Here's how the part is built. I have some questions about the finished solid (model axes, mm). A direction names the side the tool comes from. Round coordinates to 2 decimals unless told otherwise and drop trailing zeros. Write each loop counter-clockwise with the first axis right and the second up, starting at its lowest first coordinate (ties: lowest second). Pieces come first, ordered by that corner, then holes. Notation, with made-up numbers: (-30, 20.5) - (8, 20.5) arc R24 cw to (8, 57.5) - close; hole circle Ø4 at (-20.75, -32.75). An arc over 180 degrees is marked (long way). One line per question, with ' | ' between items. Start each with the question number.
(1) Will these pins go through, and if not, where does the flat tip stop? pin 1 (12 mm diameter, centred on y = -175, z = -100, fed in from +X); pin 2 (5 mm diameter, centred on x = 525, z = 23.5, fed in from +Y); pin 3 (6 mm diameter, centred on y = 211.5, z = -110.5, fed in from -X).
(2) For faces 4 (the cylindrical face through (910.575, -7.509, -23.846)), 5 (the cylindrical face through (572.9, -7.509, -23.846)), which set-ups out of +Z, -Z, +X, -X, +Y, -Y let a thin tool reach every point of the face, with its end or its side?
(3) If I drill on L1, parallel to X at y = 14.5, z = -144; L2, parallel to X at y = 77, z = -270.5; L3, parallel to Y at x = 754, z = 4.5, over which ranges is the centre line in solid material (lowest first)?
(4) Imagine slicing it at A-A (z = 84). Write out the boundary of the cut face in (x, y), plus the area to 3 significant figures.
(5) Thinking about a two-plate mould opening in X: for faces 1 (the cylindrical face through (184.875, -7.509, -23.846)), 2 (the flat face through (375, -62, 4)), 3 (the flat face through (725, -31, 2)), which applies, pulls with the +X half, pulls with the -X half, needs draft (parallel to the pull), parting line crosses it, or undercut?
(6) Imagine slicing it at D-D (z = -73.5). Write out the boundary of the cut face in (x, y).
(7) Imagine slicing it at B-B (x = 950.5). Write out the boundary of the cut face in (y, z), plus the area to 3 significant figures.
(8) Imagine slicing it at C-C (y = 240). Write out the boundary of the cut face in (x, z), plus the area to 3 significant figures.
Autodesk Inventor part; units mm, degrees
ref_plane "YZ Plane" through (0, 0, 0) normal (1, 0, 0) x (0, 1, 0)
ref_plane "XZ Plane" through (0, 0, 0) normal (0, 1, 0) x (-1, 0, 0)
ref_plane "XY Plane" through (0, 0, 0) normal (0, 0, 1) x (1, 0, 0)
sketch "Sketch1" plane through (0, 0, 0) normal (0, 1, 0) x (-1, 0, 0)
  line L0 (0, 0) -> (-400, 0) construction
  line L1 (-400, 0) -> (-750, 0)
  line L2 (-750, 0) -> (-1050, 0)
  line L3 (-400, 0) -> (-400, -300) construction
  line L4 (-400, -300) -> (-375, -300) construction
  line L5 (-375, -300) -> (-425, -300)
  line L6 (-425, -300) -> (-425, 0)
  line L7 (-425, 0) -> (-375, 0)
  line L8 (-375, 0) -> (-375, -300)
  line L9 (0, 0) -> (-1050, 0)
  line L10 (-1050, 0) -> (-1050, -25)
  line L11 (-1050, -25) -> (0, -25)
  line L12 (0, -25) -> (0, 0)
  arc A0 (0, -25) -> (25, 0) centre (0, 0) ccw
  line L13 (0, 0) -> (25, 0) construction
  line L14 (-750, 0) -> (-750, -150) construction
  line L15 (-750, -150) -> (-725, -150) construction
  line L16 (-725, -150) -> (-775, -150)
  line L17 (-775, -150) -> (-775, 0)
  line L18 (-775, 0) -> (-725, 0)
  line L19 (-725, 0) -> (-725, -150)
  arc A1 (-1075, 0) -> (-1050, -25) centre (-1050, 0) ccw
  line L20 (-1050, 0) -> (-1075, 0)
  line L21 (25, 0) -> (0, 0)
  point P0 (-775, -25)
  point P1 (-725, -25)
  point P2 (-425, -25)
  point P3 (-375, -25)
  dimension "d0" = 400
  dimension "d1" = 350
  dimension "d2" = 300
  dimension "d3" = 300
  dimension "d4" = 25
  dimension "d5" = 50
  dimension "d6" = 1050
  dimension "d7" = 25
  dimension "d8" = 150
  dimension "d9" = 25
  dimension "d10" = 50
revolve "Revolution1" add sketch "Sketch1" angle 360 about axis through (0, 0, 0) along (1, 0, 0)
sketch "Sketch2" plane through (375, 0, 0) normal (-1, 0, 0) x (0, 0, 1)
  circle A0 centre (0, 0) radius 300
  line L0 (0, 300) -> (0, 290)
  line L1 (0, 290) -> (25.5833, 307.4702)
  point P0 (14.1547, 299.6659)
  dimension "d12" = 10
extrude "Extrusion1" cut sketch "Sketch2" against normal blind 284.25 contours A0 L1 L0 picked at (7.8644, 296.5058)
sketch "Sketch3" plane through (775, 0, 0) normal (1, 0, 0) x (0, 0, -1)
  circle A0 centre (0, 0) radius 150
  line L0 (0, 150) -> (0, 140)
  line L1 (0, 140) -> (62.4254, 176.0413)
  point P0 (15.8635, 149.1588)
  dimension "d15" = 10
  dimension "d16" = 60
extrude "Extrusion2" cut sketch "Sketch3" against normal blind 139 contours A0 L1 L0 picked at (8.8167, 146.2616)
sketch "Sketch4" plane through (375, 0, 0) normal (-1, 0, 0) x (0, -0.0236, 0.9997)
  line L0 (7.0793, 299.9165) -> (-6.8433, 289.9192)
  line L1 (-6.8433, 289.9192) -> (-7.0793, 299.9165)
  arc A0 (-7.0793, 299.9165) -> (7.0793, 299.9165) centre (0, 0) ccw
  circle A1 centre (0, 0) radius 25
sketch "Sketch5" plane through (425, 0, 0) normal (1, 0, 0) x (0, 0.0236, -0.9997)
  line L0 (6.8433, 289.9192) -> (-7.0793, 299.9165)
  arc A0 (-7.0793, 299.9165) -> (7.0793, 299.9165) centre (0, 0) ccw
  line L1 (7.0793, 299.9165) -> (6.8433, 289.9192)
  circle A1 centre (0, 0) radius 25
sketch "Sketch6" plane through (725, 140, 0) normal (-1, 0, 0) x (0, 0, 1)
  line L0 (0, 0) -> (-15.8635, 9.1588)
  arc A0 (-15.8635, 9.1588) -> (0, 10) centre (0, -140) ccw
  line L1 (0, 10) -> (0, 0)
  circle A1 centre (0, -140) radius 25
sketch "Sketch7" plane through (775, 140, 0) normal (1, 0, 0) x (0, 0, -1)
  circle A0 centre (0, -140) radius 25
  line L0 (15.8635, 9.1588) -> (0, 0)
  line L1 (0, 0) -> (0, 10)
  arc A1 (0, 10) -> (15.8635, 9.1588) centre (0, -140) ccw
properties part number "shaft_model" material "Steel"
Check sheet entries:
1) pin 1: x = 425 | pin 2: y = 13.56 | pin 3: x = 375
2) face 4: +X | face 5: none
3) L1: 375 to 425, 725 to 775 | L2: 375 to 425 | L3: -149.93 to 149.93
4) outline: (375, -288) - (425, -288) - (425, 288) - (375, 288) - close; (725, -124.27) - (775, -124.27) - (775, 124.27) - (725, 124.27) - close | area: 41,200 mm^2
5) face 1: needs draft | face 2: pulls with the -X half | face 3: undercut
6) outline: (375, -290.86) - (425, -290.86) - (425, 290.86) - (375, 290.86) - close; (725, -130.76) - (775, -130.76) - (775, 130.76) - (725, 130.76) - close
7) outline: circle Ø50 at (0, 0) | area: 1,960 mm^2
8) outline: (375, -180) - (425, -180) - (425, 180) - (375, 180) - close | area: 18,000 mm^2
